```python
from build123d import *

# Parameters (mm, degrees)
F0_W     = 6.35
F0_H     = 142.875
F1_DEPTH = 38.1
F2_W     = 3.81
F2_H     = 31.75
F3_DEPTH = 6.351
F5_D     = 2.7051
F5_DEPTH = 15.0876
F5_TIP   = 0.8126940303
F8_D     = 2.7051
F8_DEPTH = 14.224
F8_TIP   = 0.8126940303
F9_D     = 2.7051
F9_DEPTH = 8.89
F9_TIP   = 0.8126940303


with BuildPart() as f1:
    # F0 (on Top) → F1 (new body)
    with BuildSketch(Plane.XY):
        Rectangle(F0_W, F0_H)
    extrude(amount=F1_DEPTH)

    # F2 (on face) → F3 (cut, through all)
    with BuildSketch(Plane(origin=(-3.175, 0, 0), x_dir=(0, -1, 0), z_dir=(-1, 0, 0))):
        with Locations((-59.69, 22.225)):
            Rectangle(F2_W, F2_H)
        with Locations((-27.94, 22.225)):
            Rectangle(F2_W, F2_H)
        with Locations((3.81, 22.225)):
            Rectangle(F2_W, F2_H)
        with Locations((35.56, 22.225)):
            Rectangle(F2_W, F2_H)
    extrude(amount=-F3_DEPTH, mode=Mode.SUBTRACT)

    # F5
    with Locations(Plane(origin=(0, 0, 0), x_dir=(1, 0, 0), z_dir=(0, 0, -1))):
        with Locations((0, 46.0375), (0, -46.0375)):
            Hole(F5_D / 2, depth=F5_DEPTH)
            with Locations((0, 0, -(F5_DEPTH + F5_TIP / 2))):  # 118° drill point
                Cone(0, F5_D / 2, F5_TIP, mode=Mode.SUBTRACT)

    # F8
    with Locations(Plane.XZ.offset(71.4375)):
        with Locations((0, 31.75), (0, 6.35)):
            Hole(F8_D / 2, depth=F8_DEPTH)
            with Locations((0, 0, -(F8_DEPTH + F8_TIP / 2))):  # 118° drill point
                Cone(0, F8_D / 2, F8_TIP, mode=Mode.SUBTRACT)

    # F9
    with Locations(Plane(origin=(0, 71.4375, 0), x_dir=(-1, 0, 0), z_dir=(0, 1, 0))):
        with Locations((0, 31.75), (0, 6.35)):
            Hole(F9_D / 2, depth=F9_DEPTH)
            with Locations((0, 0, -(F9_DEPTH + F9_TIP / 2))):  # 118° drill point
                Cone(0, F9_D / 2, F9_TIP, mode=Mode.SUBTRACT)


solid = f1.part
```
Check sheet for the modelled part. Datum: model origin and axes. Units: mm. A direction names the side the tool comes from. Give positions to 0.01 mm unless a question says otherwise; leave off trailing zeros. Order: outer loops, then holes, each group sorted by start corner. A loop starts at its lowest first (then second) coordinate and runs counter-clockwise, first axis right, second up. Notation, with made-up numbers: (60, 22.25) -> (99, 22.25) arc R24 ccw to (99, 53.25) -> close; hole circle Ø8 at (80, 38.5). An arc over 180 degrees is marked (long way). Use CSV: the item, a comma, the result in double quotes. Start each with the question number.
1) Sectioned sample at B-B, the plane z = 9.5. Record the boundary of the cut face in (x, y) (1 decimal), plus the area to 3 significant figures.
2) Material ranges on line 1 (Y direction, x = 2.5, z = 7) (1 decimal); line 2 (Y direction, x = 0, z = 4); line 3 (Z direction, x = 0, y = 67.25), recorded low to high. Write a range as from..to.
3) Go/stop test with flat-tipped pins: P1, Ø3, axis at x = 0.5, y = 28, coming from the +Z side; P2, Ø1.6, axis at x = 0, z = 31.75, coming from the +Y side; P3, Ø2, axis at x = 0, z = 31.75, coming from the +Y side. Record where each tip stops, or that it passes through.
4) Sectioned sample at A-A, the plane z = 35. Record the boundary of the cut face in (x, y) (1 decimal).
5) Set-up check for faces 4 (the face through (-0.29, 66.93, 5.03)), 5 (the face through (0, -33.655, 22)), 6 (the face through (-0.727, -47.178, 7.649)): record each of +Z, -Z, +X, -X, +Y, -Y from which the full face is reachable in a straight line by a thin tool's end or side.
6) Mould release check, pull along X, two halves, no side actions. Record for faces 1 (the face through (-3.175, -1, 19)), 2 (the face through (0, -71.438, 19)), 3 (the face through (0.031, 61.876, 6.583)): released by +X, released by -X, zero draft, split by the parting line, or undercut.
Recorded:
1,outline,"(-3.2, -71.4) -> (3.2, -71.4) -> (3.2, -37.5) -> (-3.2, -37.5) -> close; (-3.2, -33.7) -> (3.2, -33.7) -> (3.2, -5.7) -> (-3.2, -5.7) -> close; (-3.2, -1.9) -> (3.2, -1.9) -> (3.2, 26) -> (-3.2, 26) -> close; (-3.2, 29.8) -> (3.2, 29.8) -> (3.2, 57.8) -> (-3.2, 57.8) -> close; (-3.2, 61.6) -> (3.2, 61.6) -> (3.2, 71.4) -> (-3.2, 71.4) -> close; hole circle Ø2.7 at (0, -46); hole circle Ø2.7 at (0, 46)"
1,area,"799 mm2"
2,line 1,"-71.4..-37.5, -33.7..-5.7, -1.9..26, 29.8..57.8, 61.6..71.4"
2,line 2,"-71.44..-47.39, -44.68..44.68, 47.39..71.44"
2,line 3,"0..5, 7.7..30.4, 33.1..38.1"
3,P1,"z = 6.35"
3,P2,"y = 62.22"
3,P3,"y = 62.34"
4,outline,"(-3.2, -71.4) -> (3.2, -71.4) -> (3.2, -37.5) -> (-3.2, -37.5) -> close; (-3.2, -33.7) -> (3.2, -33.7) -> (3.2, -5.7) -> (-3.2, -5.7) -> close; (-3.2, -1.9) -> (3.2, -1.9) -> (3.2, 26) -> (-3.2, 26) -> close; (-3.2, 29.8) -> (3.2, 29.8) -> (3.2, 57.8) -> (-3.2, 57.8) -> close; (-3.2, 61.6) -> (3.2, 61.6) -> (3.2, 71.4) -> (-3.2, 71.4) -> close"
5,face 4,"+Y"
5,face 5,"+Z, +X, -X"
5,face 6,"-Z"
6,face 1,"released by -X"
6,face 2,"zero draft"
6,face 3,"undercut"
